Work out the finished part from the listing and answer in its coordinate system (mm). A direction names the side the tool comes from. Give positions to 0.01 mm unless a question says otherwise; leave off trailing zeros. Write each loop counter-clockwise with the first axis right and the second up, starting at its lowest first coordinate (ties: lowest second). Pieces come first, ordered by that corner, then holes. Notation, with made-up numbers: (32.5, 0.5) -> (70.5, 0.5) arc R16 cw to (70.5, 15.5) -> close; hole circle Ø7 at (-3, 25.5). An arc over 180 degrees is marked (long way). Use a Markdown table: item, result. Add a question column.
Q1. For a pull along X with two mould halves and no side action, classify faces 1 (the face through (-39.418, 22.656, 1.972)), 2 (the face through (-7.254, -39.427, 1.972)), 3 (the face through (-36, -5, 4)) as pulls with the +X half, pulls with the -X half, needs draft (parallel to the pull), parting line crosses it, or undercut.
Q2. This flat-tipped pin is pushed along its axis until it touches: pin 1 Ø3.5 at (x, y) = (-8, -47) entering from +Z. Where does it stop, or does it pass through?
Q3. Section A-A, the plane y = -12 is taken. Give the vertices of the cut face in (x, z).
Q4. Consider line 1 (X direction, y = -25, z = 0.3); line 2 (Z direction, x = -37, y = -59); line 3 (Y direction, x = -5, z = 0.25). Determine where each line is inside the solid, lowest interval first.
Q5. Section B-B, the plane z = 1.4 is taken. State how many separate pieces and enclosed holes the cut face has, plus the area to 3 significant figures.
Q6. Section C-C, the plane x = -13.5 is taken. Give the vertices of the cut face in (y, z), plus the area to 3 significant figures.
Q7. For faces 4 (the face through (-6.114, 23.604, 1.972)), 5 (the face through (-35, 15, 0.5)), determine the directions among +Z, -Z, +X, -X, +Y, -Y from which every point of the face is accessible in a straight line to the end or side of a thin tool.
from build123d import *

# Parameters (mm, degrees)
F1_DEPTH = 0.5
F0_R     = 1.8
F0_R_2   = 1.75
F0_R_3   = 1.7
F0_R_4   = 1.65
F0_R_5   = 1.45
F0_R_6   = 1.5
F0_R_7   = 1.55
F0_R_8   = 1.6
F2_DEPTH = 4
F3_SIZE  = 0.5


# Not quite as in the source:
# - a feature names something its author has since deleted; it is built from what else it names


with BuildPart() as f1:
    # F0 (on Top) → F1 (new body)
    with BuildSketch(Plane.XY):
        with BuildLine():
            ThreePointArc((-34.4459491638, 25.172913447), (-33.7578745255, 23.955043307), (-33.5192581371, 22.5767412339))
            ThreePointArc((-33.5192581371, 22.5767412339), (-35.3994402039, 19.129654298), (-39.3155548901, 18.8441044547))
            Line((-39.3155548901, 18.8441044547), (-39.3856102198, -3.8797168626))
            ThreePointArc((-39.3856102198, -3.8797168626), (-36.7220470885, -2.9687824702), (-34.1081989909, -4.0138509584))
            Line((-34.1081989909, -4.0138509584), (-34.0341191547, 20.0153980404))
            Line((-34.0341191547, 20.0153980404), (-9.9966601452, 20.0153980404))
            ThreePointArc((-9.9966601452, 20.0153980404), (-11.4744909058, 22.4082296795), (-10.9585929746, 25.172913447))
            Line((-10.9585929746, 25.172913447), (-34.4459491638, 25.172913447))
        make_face()
    extrude(amount=F1_DEPTH)



with BuildPart() as f1b:
    # F0 (on Top) → F1, piece 2 (new body)
    with BuildSketch(Plane.XY):
        with BuildLine():
            ThreePointArc((-34.1267702169, -10.0377926374), (-36.747012257, -11.0667249351), (-39.4049081675, -10.1393850024))
            Line((-39.4049081675, -10.1393850024), (-39.4799453288, -34.4791611719))
            ThreePointArc((-39.4799453288, -34.4791611719), (-36.7996355415, -33.5950156167), (-34.2028031384, -34.7005631683))
            Line((-34.2028031384, -34.7005631683), (-34.1267702169, -10.0377926374))
        make_face()
    extrude(amount=F1_DEPTH)


with BuildPart() as f1c:
    # F0 (on Top) → F1, piece 3 (new body)
    with BuildSketch(Plane.XY):
        with BuildLine():
            Line((-5.5554180266, -3.69580099), (-5.5964215167, 19.8019486813))
            ThreePointArc((-5.5964215167, 19.8019486813), (-7.6604313925, 19.2233417208), (-9.7184515138, 19.8229048634))
            Line((-9.7184515138, 19.8229048634), (-9.6771501637, -3.8455385501))
            ThreePointArc((-9.6771501637, -3.8455385501), (-7.638026651, -3.1721760384), (-5.5554180266, -3.69580099))
        make_face()
    extrude(amount=F1_DEPTH)


with BuildPart() as f1d:
    # F0 (on Top) → F1, piece 4 (new body)
    with BuildSketch(Plane.XY):
        with BuildLine():
            ThreePointArc((-34.2206804706, -40.4994267733), (-36.8242800383, -41.5889418992), (-39.4990874596, -40.6882870387))
            Line((-39.4990874596, -40.6882870387), (-39.5762478682, -65.7167801383))
            ThreePointArc((-39.5762478682, -65.7167801383), (-36.9756537231, -64.6039381296), (-34.2978020361, -65.515320369))
            Line((-34.2978020361, -65.515320369), (-34.2206804706, -40.4994267733))
        make_face()
    extrude(amount=F1_DEPTH)


with BuildPart() as f1e:
    # F0 (on Top) → F1, piece 5 (new body)
    with BuildSketch(Plane.XY):
        with BuildLine():
            ThreePointArc((-5.5438297262, -10.3366742508), (-7.6245982257, -10.8675642808), (-9.6660593434, -10.2013223749))
            Line((-9.6660593434, -10.2013223749), (-9.6222940519, -35.2817694502))
            ThreePointArc((-9.6222940519, -35.2817694502), (-7.6890371511, -34.2390892716), (-5.5017688296, -34.440388773))
            Line((-5.5017688296, -34.440388773), (-5.5438297262, -10.3366742508))
        make_face()
    extrude(amount=F1_DEPTH)


with BuildPart() as f1f:
    # F0 (on Top) → F1, piece 6 (new body)
    with BuildSketch(Plane.XY):
        with BuildLine():
            ThreePointArc((-5.4894862388, -41.4791369772), (-7.6760387081, -41.6880687805), (-9.6129227708, -40.6521419841))
            Line((-9.6129227708, -40.6521419841), (-9.5691439378, -65.7403492338))
            ThreePointArc((-9.5691439378, -65.7403492338), (-7.5101002942, -65.1167253071), (-5.4471731405, -65.7273799451))
            Line((-5.4471731405, -65.7273799451), (-5.4894862388, -41.4791369772))
        make_face()
    extrude(amount=F1_DEPTH)


with BuildPart() as f1_1:
    add(f1.part)

    add(f1b.part)  # F2 merges F1b

    add(f1c.part)  # F2 merges F1c

    add(f1d.part)  # F2 merges F1d

    add(f1e.part)  # F2 merges F1e

    add(f1f.part)  # F2 merges F1f
    # F0 (on Top) → F2 (join)
    with BuildSketch(Plane.XY):
        with BuildLine():
            ThreePointArc((-39.3155548901, 18.8441044547), (-35.3994402039, 19.129654298), (-33.5192581371, 22.5767412339))
            ThreePointArc((-33.5192581371, 22.5767412339), (-33.7578745255, 23.955043307), (-34.4459491638, 25.172913447))
            ThreePointArc((-34.4459491638, 25.172913447), (-40.8686961023, 25.0769718053), (-39.3155548901, 18.8441044547))
        make_face()
        with Locations((-37.6192581371, 22.5767412339)):
            Circle(F0_R, mode=Mode.SUBTRACT)
        with BuildLine():
            ThreePointArc((-34.1081989909, -4.0138509584), (-36.7220470885, -2.9687824702), (-39.3856102198, -3.8797168626))
            ThreePointArc((-39.3856102198, -3.8797168626), (-40.8749320279, -7.0049892451), (-39.4049081675, -10.1393850024))
            ThreePointArc((-39.4049081675, -10.1393850024), (-36.747012257, -11.0667249351), (-34.1267702169, -10.0377926374))
            ThreePointArc((-34.1267702169, -10.0377926374), (-33.1283221824, -8.6719940136), (-32.774951274, -7.0174749417))
            ThreePointArc((-32.774951274, -7.0174749417), (-33.1232390521, -5.3743600258), (-34.1081989909, -4.0138509584))
        make_face()
        with Locations((-36.824951274, -7.0174749417)):
            Circle(F0_R_2, mode=Mode.SUBTRACT)
        with BuildLine():
            ThreePointArc((-34.2028031384, -34.7005631683), (-36.7996355415, -33.5950156167), (-39.4799453288, -34.4791611719))
            ThreePointArc((-39.4799453288, -34.4791611719), (-40.9672886463, -37.5791682773), (-39.4990874596, -40.6882870387))
            ThreePointArc((-39.4990874596, -40.6882870387), (-36.8242800383, -41.5889418992), (-34.2206804706, -40.4994267733))
            ThreePointArc((-34.2206804706, -40.4994267733), (-33.2939911195, -39.1747703785), (-32.9673076548, -37.5914998294))
            ThreePointArc((-32.9673076548, -37.5914998294), (-33.2891275297, -36.0195612278), (-34.2028031384, -34.7005631683))
        make_face()
        with Locations((-36.9673076548, -37.5914998294)):
            Circle(F0_R_3, mode=Mode.SUBTRACT)
        with BuildLine():
            ThreePointArc((-34.2978020361, -65.515320369), (-36.9756537231, -64.6039381296), (-39.5762478682, -65.7167801383))
            ThreePointArc((-39.5762478682, -65.7167801383), (-38.363689229, -72.18905184), (-32.8750057563, -68.5510643234))
            ThreePointArc((-32.8750057563, -68.5510643234), (-33.2483484695, -66.8747521053), (-34.2978020361, -65.515320369))
        make_face()
        with Locations((-36.8250057563, -68.5510643234)):
            Circle(F0_R_4, mode=Mode.SUBTRACT)
        with BuildLine():
            ThreePointArc((-5.4471731405, -65.7273799451), (-7.5101002942, -65.1167253071), (-9.5691439378, -65.7403492338))
            ThreePointArc((-9.5691439378, -65.7403492338), (-9.2726802717, -72.1703531716), (-3.7483014256, -68.8667067453))
            ThreePointArc((-3.7483014256, -68.8667067453), (-4.2002541951, -67.0819422046), (-5.4471731405, -65.7273799451))
        make_face()
        with Locations((-7.4983014256, -68.8667067453)):
            Circle(F0_R_5, mode=Mode.SUBTRACT)
        with BuildLine():
            ThreePointArc((-5.5017688296, -34.440388773), (-7.6890371511, -34.2390892716), (-9.6222940519, -35.2817694502))
            ThreePointArc((-9.6222940519, -35.2817694502), (-10.7287867634, -37.9688947195), (-9.6129227708, -40.6521419841))
            ThreePointArc((-9.6129227708, -40.6521419841), (-7.6760387081, -41.6880687805), (-5.4894862388, -41.4791369772))
            ThreePointArc((-5.4894862388, -41.4791369772), (-3.7736884319, -40.0801206812), (-3.1287925489, -37.962263743))
            ThreePointArc((-3.1287925489, -37.962263743), (-3.7773888828, -35.8389043921), (-5.5017688296, -34.440388773))
        make_face()
        with Locations((-6.9287925489, -37.962263743)):
            Circle(F0_R_6, mode=Mode.SUBTRACT)
        with BuildLine():
            ThreePointArc((-3.6482529968, -7.0196379713), (-4.1589106487, -5.1035762076), (-5.5554180266, -3.69580099))
            ThreePointArc((-5.5554180266, -3.69580099), (-7.638026651, -3.1721760384), (-9.6771501637, -3.8455385501))
            ThreePointArc((-9.6771501637, -3.8455385501), (-11.3482471352, -7.0263561975), (-9.6660593434, -10.2013223749))
            ThreePointArc((-9.6660593434, -10.2013223749), (-7.6245982257, -10.8675642808), (-5.5438297262, -10.3366742508))
            ThreePointArc((-5.5438297262, -10.3366742508), (-4.155572217, -8.9298696861), (-3.6482529968, -7.0196379713))
        make_face()
        with Locations((-7.4982529968, -7.0196379713)):
            Circle(F0_R_7, mode=Mode.SUBTRACT)
        with BuildLine():
            ThreePointArc((-3.7406042554, 23.1232913211), (-6.5752770767, 26.8749680133), (-10.9585929746, 25.172913447))
            ThreePointArc((-10.9585929746, 25.172913447), (-11.4744909058, 22.4082296795), (-9.9966601452, 20.0153980404))
            ThreePointArc((-9.9966601452, 20.0153980404), (-9.8596440675, 19.9161333406), (-9.7184515138, 19.8229048634))
            ThreePointArc((-9.7184515138, 19.8229048634), (-7.6604313925, 19.2233417208), (-5.5964215167, 19.8019486813))
            ThreePointArc((-5.5964215167, 19.8019486813), (-4.2360255237, 21.2209654658), (-3.7406042554, 23.1232913211))
        make_face()
        with Locations((-7.6406042554, 23.1232913211)):
            Circle(F0_R_8, mode=Mode.SUBTRACT)
    extrude(amount=F2_DEPTH)

    # F3
    f3_edges = [f1_1.edges().sort_by_distance(p)[0] for p in [
        (-41.719258, 22.576741, 4),
        (-34.244994, -3.895565, 4),
        (-34.45467, -40.703838, 4),
        (-34.073764, -71.385349, 4),
        (-11.540604, 23.123291, 4),
        (-9.441088, -10.343475, 4),
        (-8.355816, -41.484139, 4),
        (-9.54943, -72.006034, 4),
    ]]
    chamfer(f3_edges, length=F3_SIZE)


solid = f1_1.part
Result set:
| question | item | result |
|---|---|---|
| 1 | face 1 | undercut |
| 1 | face 2 | undercut |
| 1 | face 3 | needs draft |
| 2 | pin 1 | stops at z = 0.5 |
| 3 | outline | (-39.41, 0) -> (-34.13, 0) -> (-34.13, 0.5) -> (-39.41, 0.5) -> close; (-9.66, 0) -> (-5.54, 0) -> (-5.54, 0.5) -> (-9.66, 0.5) -> close |
| 4 | line 1 | x = -39.45 to -34.17, -9.64 to -5.52 |
| 4 | line 2 | z = 0 to 0.5 |
| 4 | line 3 | y = -71.66 to -66.07, -41.24 to -34.69, -9.95 to -4.09, 20.25 to 25.99 |
| 5 | separate pieces | 8 |
| 5 | enclosed holes | 8 |
| 5 | area | 321 mm2 |
| 6 | outline | (20.02, 0) -> (25.17, 0) -> (25.17, 0.5) -> (20.02, 0.5) -> close |
| 6 | area | 2.58 mm2 |
| 7 | face 4 | +Z, -Z |
| 7 | face 5 | +Z |
